Source: CAD feature listing. Evaluate the final solid. Frame: model axes, mm. A direction names the side the tool comes from. Coordinates: 2 decimals unless noted, no trailing zeros. Order: outer loops, then holes, each group sorted by start corner. A loop starts at its lowest first (then second) coordinate and runs counter-clockwise, first axis right, second up.
```python
from build123d import *

# Parameters (mm, degrees)
F0_W         = 17.53
F0_H         = 10
F1_DEPTH     = 5
F3_DEPTH     = 10.001
F4_R         = 1.25
F5_DEPTH     = 10.001
F6_R         = 2.6
F7_DEPTH     = 3.5
F8_R         = 2.6
F9_DEPTH     = 3.5
F10_W        = 14.03
F10_H        = 3
F11_DEPTH    = 5.001
F12_R        = 1.2
F13_DEPTH    = 10
F14_R        = 0.5
F16_DEPTH    = 5.001
F17_T1_DEPTH = 3
F18_R        = 1
F19_DEPTH    = 10.001


# Not quite as in the source:
# - a fillet or chamfer that OpenCascade refuses, or shapes differently, is made with other operations: its cross-section is extruded or revolved along the edge and cut away or added


with BuildPart() as f1:
    # F0 (on Top) → F1 (new body)
    with BuildSketch(Plane.XY):
        Rectangle(F0_W, F0_H)
    extrude(amount=-F1_DEPTH)

    # F2 (on face) → F3 (cut, through all)
    with BuildSketch(Plane.XZ.offset(5)):
        with BuildLine():
            Line((8.765, 0), (6.265, 0))
            ThreePointArc((6.265, 0), (8.032766953, -0.732233047), (8.765, -2.5))
            Line((8.765, -2.5), (8.765, 0))
        make_face()
        with BuildLine():
            Line((8.765, -5), (8.765, -2.5))
            ThreePointArc((8.765, -2.5), (8.032766953, -4.267766953), (6.265, -5))
            Line((6.265, -5), (8.765, -5))
        make_face()
        with BuildLine():
            ThreePointArc((-6.265, -5), (-8.032766953, -4.267766953), (-8.765, -2.5))
            Line((-8.765, -2.5), (-8.765, -5))
            Line((-8.765, -5), (-6.265, -5))
        make_face()
        with BuildLine():
            ThreePointArc((-8.765, -2.5), (-8.032766953, -0.732233047), (-6.265, 0))
            Line((-6.265, 0), (-8.765, 0))
            Line((-8.765, 0), (-8.765, -2.5))
        make_face()
    extrude(amount=-F3_DEPTH, mode=Mode.SUBTRACT)

    # F4 (on face) → F5 (cut, through all)
    with BuildSketch(Plane(origin=(0, 5, 0), x_dir=(-1, 0, 0), z_dir=(0, 1, 0))):
        with Locations((6.265, -2.5)):
            Circle(F4_R)
    extrude(amount=-F5_DEPTH, mode=Mode.SUBTRACT)

    # F6 (on face) → F7 (cut)
    with BuildSketch(Plane(origin=(0, 5, 0), x_dir=(-1, 0, 0), z_dir=(0, 1, 0))):
        with Locations((-6.265, -2.5)):
            Circle(F6_R)
    extrude(amount=-F7_DEPTH, mode=Mode.SUBTRACT)

    # F8 (on face) → F9 (cut)
    with BuildSketch(Plane.XZ.offset(5)):
        with Locations((6.265, -2.5)):
            Circle(F8_R)
    extrude(amount=-F9_DEPTH, mode=Mode.SUBTRACT)

    # F10 (on face) → F11 (cut, through all)
    with BuildSketch(Plane.XY):
        with Locations((-4.25, 0)):
            Rectangle(F10_W, F10_H)
    extrude(amount=-F11_DEPTH, mode=Mode.SUBTRACT)

    # F12 (on face) → F13 (join)
    with BuildSketch(Plane(origin=(0, 5, 0), x_dir=(-1, 0, 0), z_dir=(0, 1, 0))):
        with Locations((-6.265, -2.5)):
            Circle(F12_R)
    extrude(amount=-F13_DEPTH)

    # F14
    f14_edges = [f1.edges().sort_by_distance(p)[0] for p in [
        (5.550857, 3.25, 0),
        (5.550857, -3.25, 0),
        (5.550857, -3.25, -5),
        (5.550857, 3.25, -5),
    ]]
    fillet(f14_edges, radius=F14_R)

    # F15 (on face) → F16 (cut, through all)
    with BuildSketch(Plane(origin=(0, 0, -5), x_dir=(1, 0, 0), z_dir=(0, 0, -1))):
        Polygon((8, 2.4762265265), (8, 5.5), (4.8, 5.5), (4.8, 2.5), (7.8, 1.5), align=None)
        Polygon((4.8, -5.5), (8, -5.5), (8, -2.4762265265), (7.8, -1.5), (4.8, -2.5), align=None)
    extrude(amount=-F16_DEPTH, mode=Mode.SUBTRACT)

    # F17: fillet of radius 2.5 on 2 edges, made by hand

    # F17_s2 → F17_t1 (cut)
    with BuildSketch(Plane.XZ.offset(-1.5)):
        with BuildLine():
            ThreePointArc((2.765, -2.5), (3.497233047, -0.732233047), (5.265, 0))
            Line((5.265, 0), (2.765, 0))
            Line((2.765, 0), (2.765, -2.5))
        make_face()
        with BuildLine():
            ThreePointArc((2.765, -2.5), (3.497233047, -4.267766953), (5.265, -5))
            Line((5.265, -5), (2.765, -5))
            Line((2.765, -5), (2.765, -2.5))
        make_face()
    extrude(amount=F17_T1_DEPTH, mode=Mode.SUBTRACT)

    # F18 (on face) → F19 (cut, through all)
    with BuildSketch(Plane.XZ.offset(5)):
        with Locations((0, -2.5)):
            Circle(F18_R)
    extrude(amount=-F19_DEPTH, mode=Mode.SUBTRACT)


solid = f1.part
```
1. Pin query (flat end, axial travel): P1, Ø1.5, axis at x = -6.265, z = -2.5, coming from the -Y side; P2, Ø2, axis at y = -3, z = -4.5, coming from the -X side. Return the tip coordinate at first contact, or that it passes through.
Findings:
P1: passes through
P2: stops at x = -8.56
2. Section query D-D on z = -2.2. Count the separate pieces of the cut face and the enclosed holes in it, plus the area to 3 significant figures.
Findings:
separate pieces: 5
enclosed holes: 0
area: 76.9 mm2
3. Ray query, line 1 (Z direction, x = 0, y = -2.6); line 2 (Y direction, x = -3.25, z = -0.4); line 3 (X direction, y = -2.5, z = -2.9). Return the intervals inside material, ascending.
Findings:
line 1: z = -5 to -3.5, -1.5 to 0
line 2: y = -5 to -1.5, 1.5 to 5
line 3: x = -8.73 to -7.45, -5.08 to -0.92, 0.92 to 3.7
4. Section query B-B on y = 3.5. Return loops of the section in (x, z) (3 decimals), plus the area to 3 significant figures.
Findings:
outline: (-6.265, -5) - (3.896, -5) arc R0.5 ccw to (4.278, -4.177) arc R2.6 cw to (4.278, -0.823) arc R0.5 ccw to (3.896, 0) - (-6.265, 0) arc R2.5 ccw to start; hole circle Ø2.5 at (-6.265, -2.5); hole circle Ø2 at (0, -2.5)
area: 53.1 mm2
5. Access query for faces 5 (the face through (4.347, -3.274, -0.282)), 6 (the face through (3.665, 3.274, -2.526)), 7 (the face through (5.12, -1.85, -2.14)). Directions: +Z, -Z, +X, -X, +Y, -Y. A direction counts if a zero-diameter tool reaches every point of the face in a straight line with its end or side. Return the directions, or none.
Findings:
face 5: +X, -Y
face 6: +Y
face 7: -Y
6. Draft query along Z for faces 1 (the face through (-1, 3, 0)), 2 (the face through (-7.457, 3.274, -2.125)), 3 (the face through (5.12, 1.86, -2.14)), 4 (the face through (-0.217, -3.274, -3.476)). Return one class per face: released by +Z, released by -Z, zero draft, split by the parting line, or undercut.
Findings:
face 1: released by +Z
face 2: undercut
face 3: split by the parting line
face 4: undercut
7. Section query A-A on x = 0. Return loops of the section in (y, z), plus the area to 3 significant figures.
Findings:
outline: (-5, -5) - (-1.5, -5) - (-1.5, -3.5) - (-5, -3.5) - close; (-5, -1.5) - (-1.5, -1.5) - (-1.5, 0) - (-5, 0) - close; (1.5, -5) - (5, -5) - (5, -3.5) - (1.5, -3.5) - close; (1.5, -1.5) - (5, -1.5) - (5, 0) - (1.5, 0) - close
area: 21.0 mm2
8. Section query C-C on y = -0.75. Return loops of the section in (x, z) (3 decimals).
Findings:
outline: (5.265, -5) - (6.265, -5) arc R2.5 ccw to (6.265, 0) - (5.265, 0) arc R2.5 ccw to start
